Check sheet for the modelled part. Datum: model origin and axes. Units: mm. A direction names the side the tool comes from. Round coordinates to 2 decimals unless told otherwise and drop trailing zeros. Order: outer loops, then holes, each group sorted by start corner. A loop starts at its lowest first (then second) coordinate and runs counter-clockwise, first axis right, second up.
Autodesk Inventor part; units mm, degrees
ref_plane "YZ Plane" through (0, 0, 0) normal (1, 0, 0) x (0, 1, 0)
ref_plane "XZ Plane" through (0, 0, 0) normal (0, 1, 0) x (-1, 0, 0)
ref_plane "XY Plane" through (0, 0, 0) normal (0, 0, 1) x (1, 0, 0)
sketch "Szkic1" plane through (0, 0, 0) normal (0, 0, 1) x (1, 0, 0)
  arc A0 (-20.1556, -10) -> (20.1556, -10) centre (0, 0) ccw
  line L0 (-20.1556, -10) -> (-67, -10)
  line L1 (-67, -10) -> (-67, 8)
  line L2 (-67, 8) -> (-23, 8)
  line L3 (-23, 8) -> (-23, 36)
  line L4 (-23, 36) -> (23, 36)
  line L5 (23, 36) -> (23, 8)
  line L6 (23, 8) -> (67, 8)
  line L7 (67, 8) -> (67, -10)
  line L8 (67, -10) -> (20.1556, -10)
  point P0 (0, -22.5)
  dimension "d0" = 45
  dimension "d1" = 10
  dimension "d2" = 18
  dimension "d3" = 46
  dimension "d4" = 44
  dimension "d5" = 44
  dimension "d6" = 23
  dimension "d7" = 58.5
extrude "Wyciągnięcie proste1" add sketch "Szkic1" against normal blind 50
sketch "Szkic2" plane through (0, 0, 0) normal (0, 0, 1) x (1, 0, 0)
  circle A0 centre (0, 0) radius 12.5
  dimension "d10" = 25
extrude "Wyciągnięcie proste2" cut sketch "Szkic2" against normal blind 50
sketch "Szkic3" plane through (23, 8, 0) normal (0, 1, 0) x (1, 0, 0)
  line L0 (0, 50) -> (44, 50)
  line L1 (44, 50) -> (9, 50)
  line L2 (9, 50) -> (9, 20)
  line L3 (9, 20) -> (44, 20)
  line L4 (44, 20) -> (44, 50)
  line L5 (-90, 50) -> (-46, 50)
  line L6 (-90, 50) -> (-55, 50)
  line L7 (-55, 50) -> (-55, 20)
  line L8 (-55, 20) -> (-90, 20)
  line L9 (-90, 20) -> (-90, 50)
  point P0 (-23, 0)
  point P1 (9, 50)
  dimension "d13" = 35
  dimension "d14" = 30
  dimension "d15" = 35
  dimension "d16" = 30
extrude "Wyciągnięcie proste3" add sketch "Szkic3" along normal blind 12
sketch "Szkic4" plane through (-23, 36, 0) normal (0, 1, 0) x (1, 0, 0)
  circle A0 centre (23, 77.2029) radius 42
  point P0 (23, 0)
  point P1 (-9, 50)
  point P2 (55, 50)
  dimension "d19" = 84
extrude "Wyciągnięcie proste4" cut sketch "Szkic4" against normal blind 141.25
chamfer "Faza1" distance 3 angle 45 16 edges at (-45, 8, 0) (-23, 22, 0) (-67, 8, -10) (-67, 14, -20) (-49.5, 20, -20) (-67, -1, 0) (-43.5778, -10, 0) (0, -22.5, 0) (43.5778, -10, 0) (67, -1, 0) (45, 8, 0) (23, 22, 0) (67, 8, -10) (67, 14, -20) (49.5, 20, -20) (-12.5, 0, 0)
sketch "Szkic5" plane through (0, 36, -77.2029) normal (0, 1, 0) x (1, 0, 0)
  point P0 (0, -77.2029)
  point P1 (0, -63.2029)
  point P2 (161.096, 29.7407)
  dimension "d25" = 14
hole "Otwór1" at (161.096, 36, -106.9437) at (0, 36, -14) direction (0, -1, 0) diameter 5.5 depth 23.81 tip angle 118 countersink diameter 10.4 countersink angle 90
properties part number "zad 8"
1) Set-up check for faces 1 (the face through (-22, 21, -2)), 2 (the face through (-23, 22, -22)), 3 (the face through (65, 7, -13)): record each of +Z, -Z, +X, -X, +Y, -Y from which the full face is reachable in a straight line by a thin tool's end or side.
2) Sectioned sample at A-A on x = 0. Record the cut outline in (y, z).
3) Sectioned sample at B-B on z = -5. Record the cut outline in (x, y), and give its area (3 significant figures).
4) Gauge pin test, flat ends, axial feed: pin 1 (12.5 mm diameter, centred on x = 34.5, z = -26, fed in from +Y); pin 2 (7 mm diameter, centred on x = 51, y = 12, fed in from +Z); pin 3 (2 mm diameter, centred on x = -46.5, z = -11.5, fed in from +Y). Record the tip position at first contact, or that the pin passes through.
5) Draft check along Y on faces 4 (the face through (1.673, 22.722, -16.182)), 5 (the face through (5.77, -11.09, -19.82)), 6 (the face through (44, -10, -26)), 7 (the face through (12.102, 3.811, -2.812)). Enter one of: pulls with the +Y half, pulls with the -Y half, needs draft (parallel to the pull), parting line crosses it, or undercut.
6) Sectioned sample at C-C on y = 0. Record the cut outline in (x, z), and give its area (3 significant figures).
7) Sectioned sample at D-D on x = -37.5. Record the cut outline in (y, z).
8) Scan lines: line 1 (Y direction, x = 0, z = -23); line 2 (Z direction, x = 0, y = 18.25); line 3 (X direction, y = 10, z = -29). Record each from-to range of solid material in increasing order.
Values found:
1. face 1: +Z, -X, +Y
1. face 2: +Z, -Z, +Y
1. face 3: +Z, +X, +Y
2. outline: (-22.5, -35.2) - (-12.5, -35.2) - (-12.5, -3) - (-15.5, 0) - (-19.5, 0) - (-22.5, -3) - close; (12.5, -35.2) - (36, -35.2) - (36, -19.2) - (33.55, -16.75) - (12.5, -16.75) - close; (12.5, -11.25) - (33.55, -11.25) - (36, -8.8) - (36, 0) - (15.5, 0) - (12.5, -3) - close
3. outline: (-67, -10) - (-20.16, -10) arc R22.5 ccw to (20.16, -10) - (67, -10) - (67, 5) - (64, 8) - (23, 8) - (23, 36) - (-23, 36) - (-23, 8) - (-64, 8) - (-67, 5) - close; hole circle Ø25 at (0, 0)
3. area: 3,560 mm2
4. pin 1: stops at y = 20
4. pin 2: stops at z = -20
4. pin 3: stops at y = 8
5. face 4: needs draft
5. face 5: undercut
5. face 6: pulls with the -Y half
5. face 7: undercut
6. outline: (-67, -50) - (-32, -50) arc R42 cw to (-12.5, -37.11) - (-12.5, -3) - (-15.5, 0) - (-64, 0) - (-67, -3) - close; (12.5, -37.11) arc R42 cw to (32, -50) - (67, -50) - (67, -3) - (64, 0) - (15.5, 0) - (12.5, -3) - close
6. area: 5,130 mm2
7. outline: (-10, -50) - (20, -50) - (20, -23) - (17, -20) - (8, -20) - (8, -3) - (5, 0) - (-7, 0) - (-10, -3) - close
8. line 1: y = -22.5 to -12.5, 12.5 to 36
8. line 2: z = -35.2 to -16.75, -11.25 to 0
8. line 3: x = -67 to -32, -23 to -7.5, 7.5 to 23, 32 to 67
